```python
from build123d import *

# Parameters (mm, degrees)
SKETCH1_W               = 20
SKETCH1_H               = 80
BOSS_EXTRUDE1_DEPTH     = 6.35
SKETCH2_R               = 1.55
MOTOR_MOUNT_HOLES_DEPTH = 10
SKETCH3_R               = 11.5
FLANGE_HOLE_DEPTH       = 10


with BuildPart() as part:
    # Sketch1 → Boss-Extrude1 (new body)
    with BuildSketch(Plane(origin=(0, 0, 0), x_dir=(0, 0, -1), z_dir=(1, 0, 0))):
        with Locations((-10, 40)):
            Rectangle(SKETCH1_W, SKETCH1_H)
    boss_extrude1 = extrude(amount=BOSS_EXTRUDE1_DEPTH)

    # Sketch2 → Motor Mount Holes (cut)
    with BuildSketch(Plane(origin=(6.35, 0, 0), x_dir=(0, 0, -1), z_dir=(1, 0, 0))):
        with Locations((-15.5, 5.75)):
            Circle(SKETCH2_R)
        with Locations((-15.5, 36.75)):
            Circle(SKETCH2_R)
    motor_mount_holes = extrude(amount=-MOTOR_MOUNT_HOLES_DEPTH, mode=Mode.SUBTRACT)

    # Sketch3 → Flange Hole (cut)
    with BuildSketch(Plane(origin=(6.35, 0, 0), x_dir=(0, 0, -1), z_dir=(1, 0, 0))):
        with Locations((0, 21.25)):
            Circle(SKETCH3_R)
    flange_hole = extrude(amount=-FLANGE_HOLE_DEPTH, mode=Mode.SUBTRACT)

    # Mirror1: Boss-Extrude1, Motor Mount Holes, Flange Hole across plane
    add(boss_extrude1.mirror(Plane(origin=(6.35, 0, 0), x_dir=(1, 0, 0), z_dir=(0, 0, 1))))
    add(motor_mount_holes.mirror(Plane(origin=(6.35, 0, 0), x_dir=(1, 0, 0), z_dir=(0, 0, 1))), mode=Mode.SUBTRACT)
    add(flange_hole.mirror(Plane(origin=(6.35, 0, 0), x_dir=(1, 0, 0), z_dir=(0, 0, 1))), mode=Mode.SUBTRACT)


solid = part.part
```
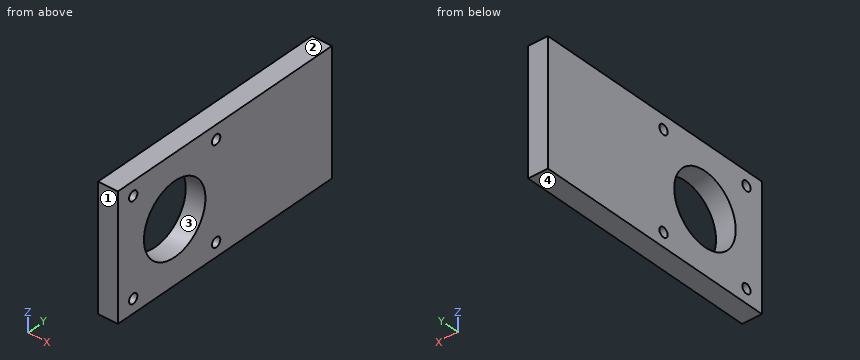
Model file for the job. Use its own axes, mm. Face numbers are marked on the shaded views. Coordinates: 2 decimals unless noted, no trailing zeros. Loops run counter-clockwise (first coordinate to the right, second up) from the corner with the lowest first, then second, coordinate; pieces in that order, holes last. Notation, with made-up numbers: (29, 7.25) - (83, 7.25) arc R20 ccw to (83, 11.25) - close; hole circle Ø1 at (-22, 87). An arc over 180 degrees is marked (long way). Write item = value, one per line. Start each with the question number.
Item 1: Saw through at D-D, the plane y = 21.25. List the corners of the cut face in (x, z).
Item 2: Pull direction Z, two halves, no side cores. Call the marked faces 1, 2, 3 and 4: +Z half, -Z half, draft (parallel to the pull), parting line (faces both ways), or undercut.
Item 3: Wall check: probe 1 along Y at (x, z) = (3.5, -15.5); probe 2 along Y at (x, z) = (2, 7); probe 3 along Y at (x, z) = (3.25, -16.5). Give the ranges that are in metal, low to high. Write a range as [from, to].
Item 4: Saw through at A-A, the plane z = 0. List the corners of the cut face in (x, y), then the cut area to 3 significant figures.
Item 5: Saw through at C-C, the plane x = 3.75. List the corners of the cut face in (y, z).
Item 6: Saw through at B-B, the plane y = 36.75. List the corners of the cut face in (x, z), then the cut area to 3 significant figures.
Answers:
q1.outline = (0, -20) - (6.35, -20) - (6.35, -11.5) - (0, -11.5) - close; (0, 11.5) - (6.35, 11.5) - (6.35, 20) - (0, 20) - close
q2.face_1 = draft
q2.face_2 = +Z half
q2.face_3 = undercut
q2.face_4 = -Z half
q3.probe_1 = [0, 4.2], [7.3, 35.2], [38.3, 80]
q3.probe_2 = [0, 12.13], [30.37, 80]
q3.probe_3 = [0, 4.57], [6.93, 35.57], [37.93, 80]
q4.outline = (0, 0) - (6.35, 0) - (6.35, 9.75) - (0, 9.75) - close; (0, 32.75) - (6.35, 32.75) - (6.35, 80) - (0, 80) - close
q4.area = 362 mm2
q5.outline = (0, -20) - (80, -20) - (80, 20) - (0, 20) - close; hole circle Ø3.1 at (5.75, -15.5); hole circle Ø3.1 at (5.75, 15.5); hole circle Ø23 at (21.25, 0); hole circle Ø3.1 at (36.75, -15.5); hole circle Ø3.1 at (36.75, 15.5)
q6.outline = (0, -20) - (6.35, -20) - (6.35, -17.05) - (0, -17.05) - close; (0, -13.95) - (6.35, -13.95) - (6.35, 13.95) - (0, 13.95) - close; (0, 17.05) - (6.35, 17.05) - (6.35, 20) - (0, 20) - close
q6.area = 215 mm2
